Geometry check sheet. Reference: drawing and pictorial views, mm from the part's lowest x, y, z. A direction names the side the tool comes from. Round coordinates to 2 decimals unless told otherwise and drop trailing zeros. Order: outer loops, then holes, each group sorted by start corner. A loop starts at its lowest first (then second) coordinate and runs counter-clockwise, first axis right, second up. Notation, with made-up numbers: (-15.5, 33) -> (22.5, 33) arc R12 ccw to (22.5, 37) -> close; hole circle Ø9 at (-40, -21.75). An arc over 180 degrees is marked (long way). Put each result on its own line as item: value.
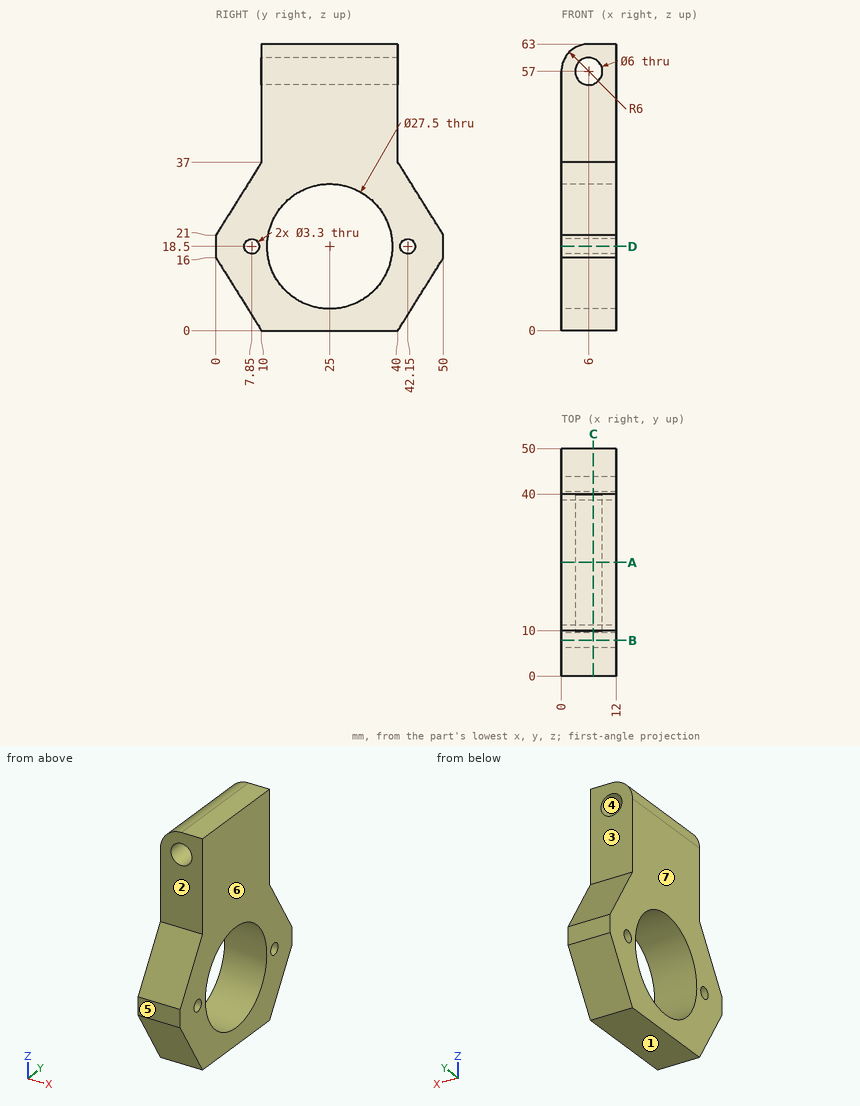
Item 1: Tool access check on the marked faces 1, 2 and 3. Record the directions out of +Z, -Z, +X, -X, +Y, -Y that give a thin tool (end or side, any length) a straight path to the whole face; none if there is none.
Geometry check:
face 1: -Z, +X, -X, +Y, -Y
face 2: +Z, +X, -X, -Y
face 3: +Z, +X, -X, +Y
Item 2: Sectioned sample at C-C, the plane x = 7. Record the boundary of the cut face in (y, z), then the cut area to 3 significant figures.
Geometry check:
outline: (0, 16) -> (10, 0) -> (40, 0) -> (50, 16) -> (50, 21) -> (40, 37) -> (40, 54.17) -> (10, 54.17) -> (10, 37) -> (0, 21) -> close; (10, 59.83) -> (40, 59.83) -> (40, 63) -> (10, 63) -> close; hole circle Ø3.3 at (7.85, 18.5); hole circle Ø27.5 at (25, 18.5); hole circle Ø3.3 at (42.15, 18.5)
area: 1,530 mm2
Item 3: Depth check by flat-ended pin: pin 1 Ø3 at (x, y) = (8.5, 10.5) entering from -Z; pin 2 Ø2 at (x, y) = (2, 8) entering from +Z. Enter the tip coordinate at first touch or a pass-through.
Geometry check:
pin 1: z = 0
pin 2: z = 35.4
Item 4: Sectioned sample at B-B, the plane y = 7.85. Record the boundary of the cut face in (x, z).
Geometry check:
outline: (0, 3.44) -> (12, 3.44) -> (12, 16.85) -> (0, 16.85) -> close; (0, 20.15) -> (12, 20.15) -> (12, 33.56) -> (0, 33.56) -> close
Item 5: Material ranges on line 1 along Z through (x, y) = (4.75, 30.5); line 2 along Z through (x, y) = (4.75, 36.5); line 3 along Y through (x, z) = (7, 60.5), recorded low to high.
Geometry check:
line 1: 0 to 5.9, 31.1 to 54.27, 59.73 to 62.87
line 2: 0 to 10.96, 26.04 to 54.27, 59.73 to 62.87
line 3: 10 to 40
Item 6: Sectioned sample at A-A, the plane y = 25. Record the boundary of the cut face in (x, z), then the cut area to 3 significant figures.
Geometry check:
outline: (0, 0) -> (12, 0) -> (12, 4.75) -> (0, 4.75) -> close; (0, 32.25) -> (12, 32.25) -> (12, 63) -> (6, 63) arc R6 ccw to (0, 57) -> close; hole circle Ø6 at (6, 57)
area: 390 mm2
Item 7: Sectioned sample at D-D, the plane z = 18.5. Record the boundary of the cut face in (x, y).
Geometry check:
outline: (0, 0) -> (12, 0) -> (12, 6.2) -> (0, 6.2) -> close; (0, 9.5) -> (12, 9.5) -> (12, 11.25) -> (0, 11.25) -> close; (0, 38.75) -> (12, 38.75) -> (12, 40.5) -> (0, 40.5) -> close; (0, 43.8) -> (12, 43.8) -> (12, 50) -> (0, 50) -> close
Item 8: Release check for a two-part mould opening along X. For the marked faces 4, 5, 6 and 7 record: pulls with the +X half, pulls with the -X half, needs draft (parallel to the pull), parting line crosses it, or undercut.
Geometry check:
face 4: undercut
face 5: needs draft
face 6: pulls with the +X half
face 7: pulls with the -X half
